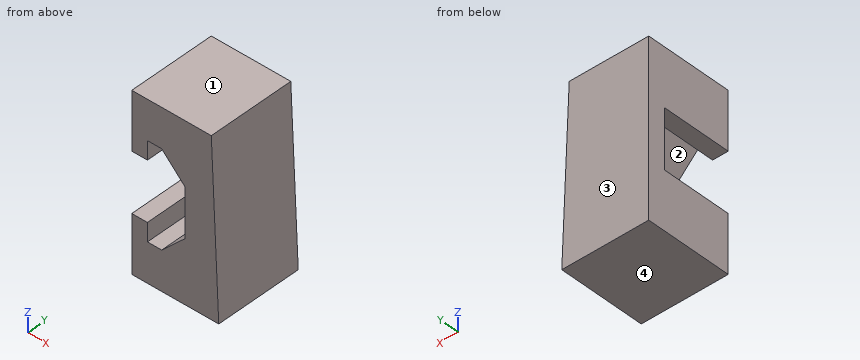
```python
from build123d import *

# Parameters (mm, degrees)
SKETCH4_W           = 10
SKETCH4_H           = 20
BOSS_EXTRUDE1_DEPTH = 10
CUT_EXTRUDE1_DEPTH  = 8
CUT_EXTRUDE2_DEPTH  = 25.494897428


with BuildPart() as part:
    # Sketch4 → Boss-Extrude1 (new body)
    with BuildSketch(Plane(origin=(0, 0, 0), x_dir=(1, 0, 0), z_dir=(0, 1, 0))):
        with Locations((5, 10)):
            Rectangle(SKETCH4_W, SKETCH4_H)
    extrude(amount=BOSS_EXTRUDE1_DEPTH)

    # Sketch2 → Cut-Extrude1 (cut)
    with BuildSketch(Plane(origin=(0, 0, 0), x_dir=(-1, 0, 0), z_dir=(0, -1, 0))):
        Polygon((0, 6.615), (-1.8, 6.615), (-1.8, 4.5), (-3.44, 4.5), (-6.1, 7.16), (-6.1, 12.84), (-3.44, 15.5), (-1.8, 15.5), (-1.8, 13.385), (0, 13.385), align=None)
    extrude(amount=-CUT_EXTRUDE1_DEPTH, mode=Mode.SUBTRACT)

    # Sketch6 → Cut-Extrude2 (cut, through all)
    with BuildSketch(Plane.XZ):
        Polygon((10, 0), (9.144267043, 0), (10, -20), align=None)
    extrude(amount=-CUT_EXTRUDE2_DEPTH, mode=Mode.SUBTRACT)


solid = part.part
```
Geometry: final body of the model. Coordinates: model frame, mm. Face numbers are marked on the shaded views. Round coordinates to 2 decimals unless told otherwise and drop trailing zeros. Order: outer loops, then holes, each group sorted by start corner. A loop starts at its lowest first (then second) coordinate and runs counter-clockwise, first axis right, second up. Notation, with made-up numbers: M 79,88.5 L 130,88.5 A11 cw 130,106.5 Z; hole C 3.5,-6 d7. An arc over 180 degrees is marked long. One line per item, written item: value.
(1) Cut plane D-D (x = 2.75). Return the cut outline in (y, z), and give its area (3 significant figures).
Result sheet:
outline: M 0,-20 L 10,-20 L 10,0 L 0,0 L 0,-4.5 L 8,-4.5 L 8,-15.5 L 0,-15.5 Z
area: 112 mm2
(2) Pin query (flat end, axial travel): P1, Ø0.6, axis at y = 4, z = -14.5, coming from the +X side; P2, Ø1.1, axis at y = 5.5, z = -6, coming from the +X side; P3, Ø1.8, axis at x = 2.5, z = -12.5, coming from the -Y side. Return the tip coordinate at first contact, or that it passes through.
Result sheet:
P1: x = 9.78
P2: x = 9.42
P3: y = 8
(3) Cut plane C-C (z = -12). Return the cut outline in (x, y), and give its area (3 significant figures).
Result sheet:
outline: M 0,8 L 6.1,8 L 6.1,0 L 9.66,0 L 9.66,10 L 0,10 Z
area: 47.8 mm2
(4) Cut plane A-A (x = 5.25). Return the cut outline in (y, z), and give its area (3 significant figures).
Result sheet:
outline: M 0,-20 L 10,-20 L 10,0 L 0,0 L 0,-6.31 L 8,-6.31 L 8,-13.69 L 0,-13.69 Z
area: 141 mm2
(5) Line query: probe 1 along Z at (x, y) = (1, 6.5) (3 decimals); probe 2 along Z at (x, y) = (2, 7.25); probe 3 along Y at (x, z) = (5.75, -9.5). Output: solid intervals per line, ascending. Write a range as [from, to].
Result sheet:
probe 1: [-20, -13.385], [-6.615, 0]
probe 2: [-20, -15.5], [-4.5, 0]
probe 3: [8, 10]
(6) Pull-direction query (Z, two-part tool) for the marked faces 1, 2, 3 and 4; classes: pulls with the +Z half, pulls with the -Z half, needs draft (parallel to the pull), parting line crosses it, or undercut.
Result sheet:
face 1: pulls with the +Z half
face 2: undercut
face 3: needs draft
face 4: pulls with the -Z half
(7) Cut plane B-B (y = 5.5). Return the cut outline in (x, z) (3 decimals).
Result sheet:
outline: M 0,-20 L 10,-20 L 9.144,0 L 0,0 L 0,-6.615 L 1.8,-6.615 L 1.8,-4.5 L 3.44,-4.5 L 6.1,-7.16 L 6.1,-12.84 L 3.44,-15.5 L 1.8,-15.5 L 1.8,-13.385 L 0,-13.385 Z
